Geometry check sheet. Reference: the model listing, model coordinates, mm. Face numbers are marked on the shaded views. A direction names the side the tool comes from. Coordinates: 2 decimals unless noted, no trailing zeros. Write each loop counter-clockwise with the first axis right and the second up, starting at its lowest first coordinate (ties: lowest second). Pieces come first, ordered by that corner, then holes. Notation, with made-up numbers: M 71,-32 L 122,-32 A4 ccw 122,-26 Z; hole C 68.5,25 d11. An arc over 180 degrees is marked long. Put each result on its own line as item: value. Start each with the question number.
1) Cross-section at C-C on x = -108. Record the cut outline in (y, z), plus the area to 3 significant figures.
2) Mould release check, pull along X, two halves, no side actions. Record for the marked faces 1 and 2: released by +X, released by -X, zero draft, split by the parting line, or undercut.
3) Cross-section at A-A on x = 94.5. Record the cut outline in (y, z), plus the area to 3 significant figures.
4) Scan lines: line 1 along Y through (x, z) = (-108, 1); line 2 along Z through (x, y) = (39.5, -36); line 3 along X through (y, z) = (-37, 109). Record each from-to range of solid material in increasing order.
5) Set-up check for the marked faces 3 and 4: record each of +Z, -Z, +X, -X, +Y, -Y from which the full face is reachable in a straight line by a thin tool's end or side.
6) Cross-section at B-B on y = -39. Record the cut outline in (x, z), plus the area to 3 significant figures.
7) Cross-section at D-D on z = 137. Record the cut outline in (x, y), plus the area to 3 significant figures.
8) Gauge pin test, flat ends, axial feed: pin 1 (12 mm diameter, centred on x = -49.5, z = 90.5, fed in from +Y); pin 2 (11 mm diameter, centred on x = -100.5, z = 4, fed in from +Y); pin 3 (1.5 mm diameter, centred on x = 77, z = 133.5, fed in from -Y). Record the tip position at first contact, or that the pin passes through.
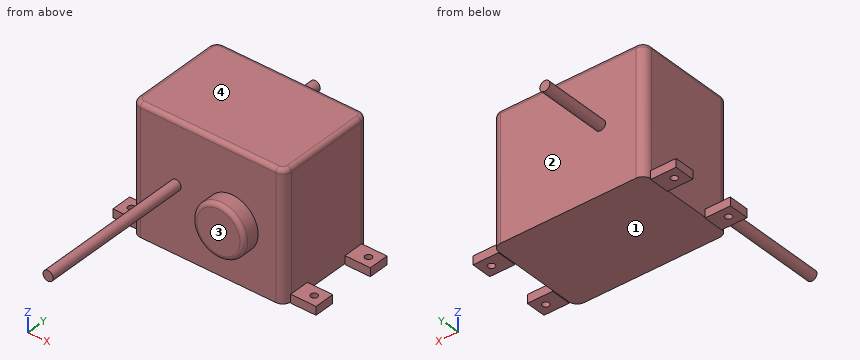
from build123d import *

# Parameters (mm, degrees)
F0_W          = 180
F0_H          = 120
F1_DEPTH      = 151
F2_R          = 10
F3_R          = 5
F5_W          = 30
F5_H          = 24
F5_R          = 4
F6_DEPTH      = 10
F7_R          = 6
F8_DEPTH      = 12.2
F9_DEPTH      = 184
F9_DEPTH_BACK = 200
F10_R         = 30.55
F10_R_2       = 6
F11_DEPTH     = 20
F12_R         = 5


with BuildPart() as f1:
    # F0 (on Top) → F1 (new body)
    with BuildSketch(Plane.XY):
        Rectangle(F0_W, F0_H)
    extrude(amount=F1_DEPTH)

    # F2
    f2_edges = [f1.edges().sort_by_distance(p)[0] for p in [
        (-90, -60, 75.5),
        (90, -60, 75.5),
        (90, 60, 75.5),
        (-90, 60, 75.5),
    ]]
    fillet(f2_edges, radius=F2_R)

    # F3
    f3_edges = [f1.edges().sort_by_distance(p)[0] for p in [
        (0, -60, 151),
    ]]
    fillet(f3_edges, radius=F3_R)

    # F5 (on offset) → F6 (join)
    with BuildSketch(Plane.XY.offset(-1)):
        with Locations((105, 39)):
            Rectangle(F5_W, F5_H)
        with Locations((108, 39)):
            Circle(F5_R, mode=Mode.SUBTRACT)
        with Locations((105, -39)):
            Rectangle(F5_W, F5_H)
        with Locations((108, -39)):
            Circle(F5_R, mode=Mode.SUBTRACT)
        with Locations((-105, -39)):
            Rectangle(F5_W, F5_H)
        with Locations((-108, -39)):
            Circle(F5_R, mode=Mode.SUBTRACT)
        with Locations((-105, 39)):
            Rectangle(F5_W, F5_H)
        with Locations((-108, 39)):
            Circle(F5_R, mode=Mode.SUBTRACT)
    extrude(amount=F6_DEPTH)

    # F7 (on face) → F8 (join)
    with BuildSketch(Plane.XZ.offset(60)):
        with Locations((38.45, 78.5)):
            Circle(F7_R)
    extrude(amount=F8_DEPTH)

    # F7 (on face) → F9 (join, two sides)
    with BuildSketch(Plane.XZ.offset(60)) as f9_sk:
        with Locations((-38, 78.5)):
            Circle(F7_R)
    extrude(amount=F9_DEPTH)
    extrude(f9_sk.sketch, amount=-F9_DEPTH_BACK)

    # F10 (on face) → F11 (join)
    with BuildSketch(Plane.XZ.offset(72.2)):
        with Locations((38.45, 78.5)):
            Circle(F10_R)
        with Locations((38.45, 78.5)):
            Circle(F10_R_2, mode=Mode.SUBTRACT)
        with Locations((38.45, 78.5)):
            Circle(F10_R_2)
    extrude(amount=F11_DEPTH)

    # F12
    f12_edges = [f1.edges().sort_by_distance(p)[0] for p in [
        (7.9, -92.2, 78.5),
    ]]
    fillet(f12_edges, radius=F12_R)


solid = f1.part
Answer key:
1. outline: M -51,-1 L -43,-1 L -43,9 L -51,9 Z; M -35,-1 L -27,-1 L -27,9 L -35,9 Z; M 27,-1 L 35,-1 L 35,9 L 27,9 Z; M 43,-1 L 51,-1 L 51,9 L 43,9 Z
1. area: 320 mm²
2. face 1: undercut
2. face 2: zero draft
3. outline: M -51,-1 L -27,-1 L -27,9 L -51,9 Z; M 27,-1 L 51,-1 L 51,9 L 27,9 Z
3. area: 480 mm²
4. line 1: y = -51 to -43, -35 to -27, 27 to 35, 43 to 51
4. line 2: z = 0 to 151
4. line 3: x = -90 to 90
5. face 3: +Z, -Z, +X, -Y
5. face 4: +Z, +X, -X, +Y, -Y
6. outline: M -120,-1 L -112,-1 L -112,9 L -120,9 Z; M -104,-1 L -90,-1 L -90,0 L 90,0 L 90,-1 L 104,-1 L 104,9 L 90,9 L 90,146 A5 ccw 85,151 L -85,151 A5 ccw -90,146 L -90,9 L -104,9 Z; M 112,-1 L 120,-1 L 120,9 L 112,9 Z
6. area: 27,600 mm²
7. outline: M -90,-50 A10 ccw -80,-60 L 80,-60 A10 ccw 90,-50 L 90,50 A10 ccw 80,60 L -80,60 A10 ccw -90,50 Z
7. area: 21,500 mm²
8. pin 1: stops at y = 60
8. pin 2: stops at y = 51
8. pin 3: stops at y = -60
